from build123d import *

# Parameters (mm, degrees)
ESQUISSE1_W        = 40
ESQUISSE1_H        = 20
BOSS_EXTRU_1_DEPTH = 40
ESQUISSE2_R        = 4.5
BOSS_EXTRU_2_DEPTH = 2
ESQUISSE3_W        = 8
ESQUISSE3_H        = 25
BOSS_EXTRU_3_DEPTH = 2
ESQUISSE4_R        = 2.5
BOSS_EXTRU_4_DEPTH = 20


with BuildPart() as part:
    # Esquisse1 → Boss.-Extru.1 (new body)
    with BuildSketch(Plane(origin=(0, 0, 0), x_dir=(1, 0, 0), z_dir=(0, 1, 0))):
        with Locations((20, 10)):
            Rectangle(ESQUISSE1_W, ESQUISSE1_H)
    extrude(amount=BOSS_EXTRU_1_DEPTH)

    # Esquisse2 → Boss.-Extru.2 (add)
    with BuildSketch(Plane(origin=(40, 0, 0), x_dir=(0, 0, -1), z_dir=(1, 0, 0))):
        with Locations(Location((10, 9.5, 0), (0, 0, 180))):
            Circle(ESQUISSE2_R)
    extrude(amount=BOSS_EXTRU_2_DEPTH)

    # Esquisse3 → Boss.-Extru.3 (add)
    with BuildSketch(Plane(origin=(0, 0, -20), x_dir=(-1, 0, 0), z_dir=(0, 0, -1))):
        with Locations((-20, 42.5)):
            Rectangle(ESQUISSE3_W, ESQUISSE3_H)
    extrude(amount=BOSS_EXTRU_3_DEPTH)

    # Esquisse4 → Boss.-Extru.4 (add)
    with BuildSketch(Plane.XY.offset(-20)):
        with Locations((20, 51)):
            Circle(ESQUISSE4_R)
    extrude(amount=BOSS_EXTRU_4_DEPTH)


solid = part.part
For this review, take the finished solid that the model builds, in its own axes (mm). A direction names the side the tool comes from. Round coordinates to 2 decimals unless told otherwise and drop trailing zeros. Write each loop counter-clockwise with the first axis right and the second up, starting at its lowest first coordinate (ties: lowest second). Pieces come first, ordered by that corner, then holes. Notation, with made-up numbers: (-38, -36) -> (-20, -36) arc R16 cw to (-20, -20) -> close; hole circle Ø7 at (-9, 31.5). An arc over 180 degrees is marked (long way). Put each result on its own line as item: value.
Q1. Consider section C-C on x = 20. State the section outline as (y, z) points, and give its area (3 significant figures).
Determined:
outline: (0, -20) -> (30, -20) -> (30, -22) -> (55, -22) -> (55, -20) -> (53.5, -20) -> (53.5, 0) -> (48.5, 0) -> (48.5, -20) -> (40, -20) -> (40, 0) -> (0, 0) -> close
area: 950 mm^2
Q2. Consider section D-D on z = -13.5. State the section outline as (x, y) points, and give its area (3 significant figures).
Determined:
outline: (0, 0) -> (40, 0) -> (40, 6.67) -> (42, 6.67) -> (42, 12.33) -> (40, 12.33) -> (40, 40) -> (0, 40) -> close; circle Ø5 at (20, 51)
area: 1,630 mm^2
Q3. Machinability: for faces 4 (the flat face through (20, 30, -21)), 5 (the flat face through (24, 42, -21)), 6 (the flat face through (20, 55, -21)), which of the approach directions +Z, -Z, +X, -X, +Y, -Y give a long, thin tool a straight path to every point of the face, cutting with its end or side? Answer none if there is none.
Determined:
face 4: -Z, +X, -X, -Y
face 5: -Z, +X, +Y, -Y
face 6: +Z, -Z, +X, -X, +Y
Q4. To check wall thickness, follow L1, parallel to Y at x = 13, z = -10; L2, parallel to Z at x = 22, y = 7. State the ranges of each line that lie inside material, in increasing order. Write a range as [from, to].
Determined:
L1: y = [0, 40]
L2: z = [-20, 0]
Q5. The part is to be moulded in two halves that separate along Y. For faces 1 (the cylindrical face through (17.5, 51.1, -10.1)), 2 (the flat face through (16, 42, -21)), 3 (the cylindrical face through (40.986, 8.148, -5.708)), say which applies: released by +Y, released by -Y, zero draft, split by the parting line, or undercut.
Determined:
face 1: undercut
face 2: zero draft
face 3: split by the parting line
Q6. Consider section B-B on y = 9.5. State the section outline as (x, z) points.
Determined:
outline: (0, -20) -> (40, -20) -> (40, -14.5) -> (42, -14.5) -> (42, -5.5) -> (40, -5.5) -> (40, 0) -> (0, 0) -> close
Q7. Clearance check with flat-ended pins moving along their axes: pin 1 Ø1 at (x, z) = (19, -10) entering from +Y; pin 2 Ø10 at (y, z) = (25.5, -10.5) entering from +X; pin 3 Ø1.6 at (y, z) = (46.5, -21) entering from -X. State where each tip first meets the part, or that it passes through.
Determined:
pin 1: stops at y = 53.45
pin 2: stops at x = 40
pin 3: stops at x = 16
Q8. Consider section A-A on z = -10. State the section outline as (x, y) points, and give its area (3 significant figures).
Determined:
outline: (0, 0) -> (40, 0) -> (40, 5) -> (42, 5) -> (42, 14) -> (40, 14) -> (40, 40) -> (0, 40) -> close; circle Ø5 at (20, 51)
area: 1,640 mm^2
